```python
from build123d import *

# Parameters (mm, degrees)
F1_DEPTH = 20
F2_R     = 4.25
F3_DEPTH = 10


with BuildPart() as f1:
    # F0 (on Top) → F1 (new body)
    with BuildSketch(Plane.XY):
        Polygon((3.257158, 63.029949), (0.257158, 63.029949), (0.257158, 54.029949), (3.257158, 54.029949), (3.257158, 58.029949), (11.757158, 58.029949), (11.757158, 8.029949), (3.257158, 8.029949), (3.257158, 12.029949), (0.257158, 12.029949), (0.257158, 3.029949), (3.257158, 3.029949), (20.257158, 3.029949), (20.257158, 27.029949), (32.257158, 27.029949), (32.257158, 39.029949), (20.257158, 39.029949), (20.257158, 63.029949), align=None)
    extrude(amount=F1_DEPTH)

    # F2 (on face) → F3 (cut)
    with BuildSketch(Plane.XY.offset(20)):
        with Locations((26.257158, 33.029949)):
            Circle(F2_R)
    extrude(amount=-F3_DEPTH, mode=Mode.SUBTRACT)


solid = f1.part
```
For this review, take the finished solid that the model builds, in its own axes (mm). A direction names the side the tool comes from. Coordinates: 2 decimals unless noted, no trailing zeros. Loops run counter-clockwise (first coordinate to the right, second up) from the corner with the lowest first, then second, coordinate; pieces in that order, holes last.
1. For faces 1 (the flat face through (2, 54.03, 10)), 2 (the flat face through (20.257, 15, 10)), 3 (the cylindrical face through (25.704, 37.244, 15.07)), list the 3-axis set-ups (+Z, -Z, +X, -X, +Y, -Y) from which the entire face can be reached by the end or side of a thin tool; tool diameter is ignored.
2. Add section C-C, the plane z = 5.5. Give the boundary of the cut face in (x, y), then the cut area to 3 significant figures.
3. For line 1 (Y direction, x = 6, z = 5.25); line 2 (Y direction, x = 21.5, z = 15.5); line 3 (X direction, y = 48.5, z = 11.25), list the stretches that pass through material, from the lowest coordinate up.
4. Add section D-D, the plane z = 12. Give the boundary of the cut face in (x, y).
5. Add section A-A, the plane y = 10.5. Give the boundary of the cut face in (x, z).
6. Add section B-B, the plane x = 11. Give the boundary of the cut face in (y, z).
7. Insertion check: P1, Ø6, axis at y = 24.5, z = 7, coming from the -X side; P2, Ø1, axis at y = 40.5, z = 12.5, coming from the +X side; P3, Ø2.5, axis at x = 25, y = 34, coming from the +Z side; P4, Ø5, axis at x = 17.5, y = 46.5, coming from the -Z side. Each pin has a flat end and moves straight along its axis. Give the tip position at first contact, or say it passes through.
8. Mouldability with a two-part tool opening along Y and no side actions: class faces 4 (the flat face through (11.757, 33, 10)), 5 (the flat face through (3.257, 10, 10)), 6 (the flat face through (26, 27.03, 10)), 7 (the flat face through (0.257, 8, 10)) as +Y half, -Y half, draft (parallel to the pull), parting line (faces both ways), or undercut.
Result:
1. face 1: +Z, -Z, -X
1. face 2: +Z, -Z, +X, -Y
1. face 3: +Z
2. outline: (0.26, 3.03) - (20.26, 3.03) - (20.26, 27.03) - (32.26, 27.03) - (32.26, 39.03) - (20.26, 39.03) - (20.26, 63.03) - (0.26, 63.03) - (0.26, 54.03) - (3.26, 54.03) - (3.26, 58.03) - (11.76, 58.03) - (11.76, 8.03) - (3.26, 8.03) - (3.26, 12.03) - (0.26, 12.03) - close
2. area: 793 mm2
3. line 1: y = 3.03 to 8.03, 58.03 to 63.03
3. line 2: y = 27.03 to 39.03
3. line 3: x = 11.76 to 20.26
4. outline: (0.26, 3.03) - (20.26, 3.03) - (20.26, 27.03) - (32.26, 27.03) - (32.26, 39.03) - (20.26, 39.03) - (20.26, 63.03) - (0.26, 63.03) - (0.26, 54.03) - (3.26, 54.03) - (3.26, 58.03) - (11.76, 58.03) - (11.76, 8.03) - (3.26, 8.03) - (3.26, 12.03) - (0.26, 12.03) - close; hole circle Ø8.5 at (26.26, 33.03)
5. outline: (0.26, 0) - (3.26, 0) - (3.26, 20) - (0.26, 20) - close; (11.76, 0) - (20.26, 0) - (20.26, 20) - (11.76, 20) - close
6. outline: (3.03, 0) - (8.03, 0) - (8.03, 20) - (3.03, 20) - close; (58.03, 0) - (63.03, 0) - (63.03, 20) - (58.03, 20) - close
7. P1: stops at x = 11.76
7. P2: stops at x = 20.26
7. P3: stops at z = 10
7. P4: stops at z = 0
8. face 4: undercut
8. face 5: undercut
8. face 6: -Y half
8. face 7: draft
